Geometry: see drawing. Coordinates: mm, zero at the bounding-box minimum. Round coordinates to 2 decimals unless told otherwise and drop trailing zeros. Order: outer loops, then holes, each group sorted by start corner. A loop starts at its lowest first (then second) coordinate and runs counter-clockwise, first axis right, second up. Notation, with made-up numbers: (-35.5, -13) -> (-19.5, -13) arc R27 cw to (-19.5, 10) -> close; hole circle Ø11 at (9, -14). An arc over 180 degrees is marked (long way). Write item = value, one per line. Start each with the question number.
(1) Ray query, line 1 (X direction, y = 1.2, z = 84.5); line 2 (X direction, y = 8.25, z = 92); line 3 (Z direction, x = 109, y = 4.5). Return the intervals inside material, ascending.
(2) Cut plane B-B on z = 84.5. Return the cut outline in (x, y), then the cut area to 3 significant figures.
(3) Cut plane C-C on x = 57.75. Return the cut outline in (y, z).
(4) Cut plane A-A on y = 3.5. Return the cut outline in (x, z).
(5) Contact query for flat-ended pins moving along their axis: pin 1 Ø1 at (x, z) = (78.5, 37.5) entering from +Y; pin 2 Ø2.5 at (x, y) = (89.5, 6) entering from -Z; pin 3 Ø3 at (x, z) = (57.75, 20.5) entering from +Y; pin 4 Ø4.5 at (x, y) = (86.5, 6) entering from +Z. Output: stop coordinate, or through.
(6) Cut plane D-D on z = 20.5. Return the cut outline in (x, y), then the cut area to 3 significant figures.
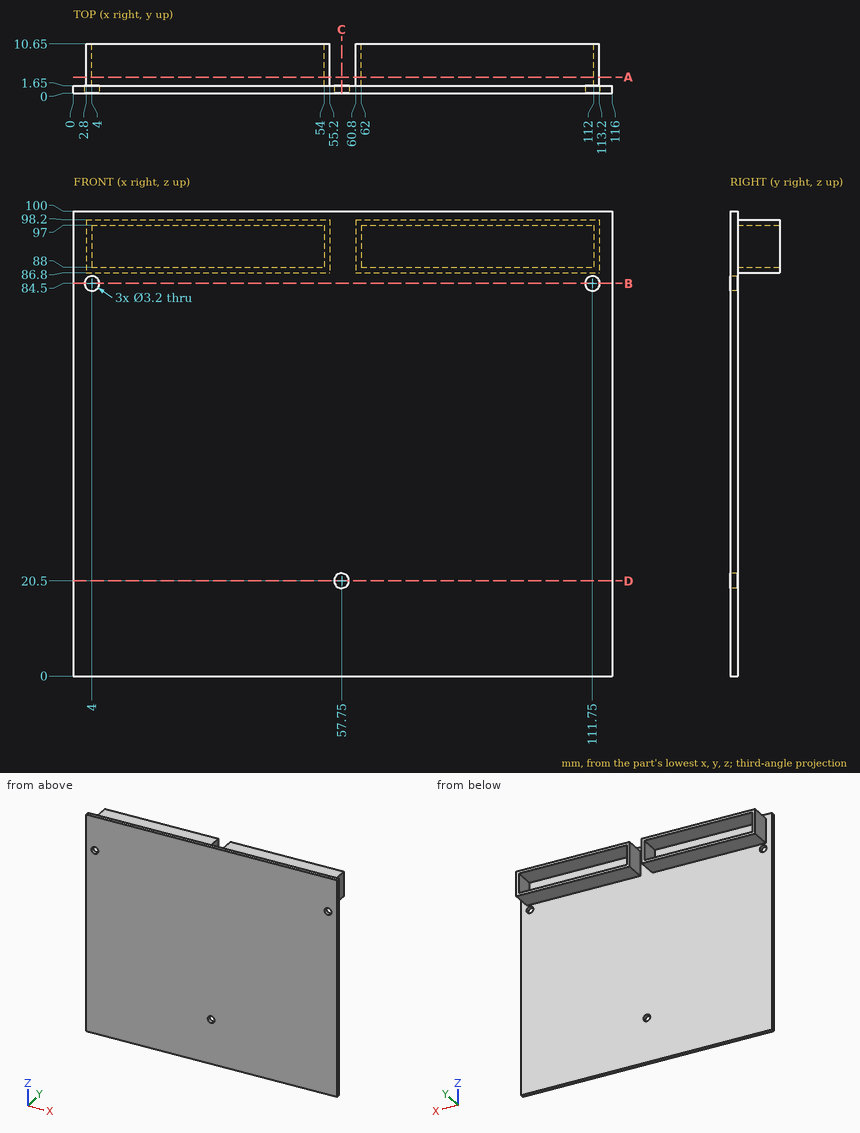
Evaluation:
q1.line_1 = 0 to 2.4, 5.6 to 110.15, 113.35 to 116
q1.line_2 = 2.8 to 4, 54 to 55.2, 60.8 to 62, 112 to 113.2
q1.line_3 = 86.8 to 88, 97 to 98.2
q2.outline = (0, 0) -> (2.4, 0) -> (2.4, 1.65) -> (0, 1.65) -> close; (5.6, 0) -> (110.15, 0) -> (110.15, 1.65) -> (5.6, 1.65) -> close; (113.35, 0) -> (116, 0) -> (116, 1.65) -> (113.35, 1.65) -> close
q2.area = 181 mm^2
q3.outline = (0, 0) -> (1.65, 0) -> (1.65, 18.9) -> (0, 18.9) -> close; (0, 22.1) -> (1.65, 22.1) -> (1.65, 100) -> (0, 100) -> close
q4.outline = (2.8, 86.8) -> (55.2, 86.8) -> (55.2, 98.2) -> (2.8, 98.2) -> close; (60.8, 86.8) -> (113.2, 86.8) -> (113.2, 98.2) -> (60.8, 98.2) -> close; hole (4, 88) -> (54, 88) -> (54, 97) -> (4, 97) -> close; hole (62, 88) -> (112, 88) -> (112, 97) -> (62, 97) -> close
q5.pin_1 = 1.65
q5.pin_2 = 86.8
q5.pin_3 = through
q5.pin_4 = 98.2
q6.outline = (0, 0) -> (56.15, 0) -> (56.15, 1.65) -> (0, 1.65) -> close; (59.35, 0) -> (116, 0) -> (116, 1.65) -> (59.35, 1.65) -> close
q6.area = 186 mm^2
